Part model, mm, in its own coordinate system. Face numbers are marked on the shaded views. A direction names the side the tool comes from. Give positions to 0.01 mm unless a question says otherwise; leave off trailing zeros. Order: outer loops, then holes, each group sorted by start corner. A loop starts at its lowest first (then second) coordinate and runs counter-clockwise, first axis right, second up.
1. Drop flat-ended pins along their axis: pin 1 Ø1.5 at (x, z) = (42, 3.5) entering from +Y; pin 2 Ø2.5 at (y, z) = (64.5, 93.5) entering from -X; pin 3 Ø3 at (y, z) = (50, 36) entering from +X. Give the stop position or say it passes through.
2. Slice it at B-B on x = 56. List the corners of the cut face in (y, z), and give its area (3 significant figures).
3. Which spindle directions (+Z, -Z, +X, -X, +Y, -Y) get a long thin tool onto all of the face, cutting with end or side? Do the marked faces 4, 5 and 6. Say none if no direction does.
4. Probe line 1 (Z direction, x = 44.5, y = 51.5); line 2 (X direction, y = 27, z = 35). List the from-to ranges inside material, lowest first.
5. Slice it at C-C on z = 46.5. List the corners of the cut face in (x, y), and give its area (3 significant figures).
6. Slice it at D-D on y = 27. List the corners of the cut face in (x, z).
7. Mould opens along Z. For the marked faces 1, 2 and 3 say: +Z half, -Z half, draft (parallel to the pull), parting line (faces both ways), or undercut.
8. Slice it at A-A on y = 58. List the corners of the cut face in (x, z).
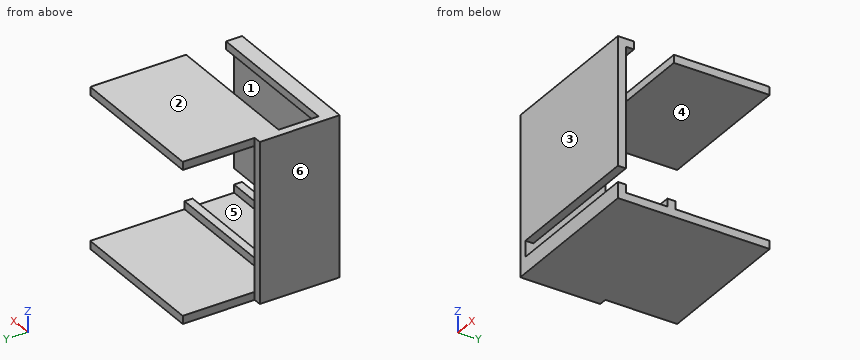
from build123d import *

# Parameters (mm, degrees)
F3_W     = 50
F3_H     = 100
F4_DEPTH = 5
F0_W     = 5
F0_H     = 5
F2_W     = 60
F2_H     = 5
F5_DEPTH = 90
F6_ANGLE = 90
F7_ANGLE = 90


with BuildPart() as f4:
    # F3 (on Top) → F4 (new body)
    with BuildSketch(Plane.XY):
        with Locations((25, 50)):
            Rectangle(F3_W, F3_H)
    extrude(amount=-F4_DEPTH)

    # F0 (on Top) + F1 (on Top) + F2 (on Top) → F5 (join)
    with BuildSketch(Plane.XY):
        Polygon((0, 10), (0, 0), (95, 0), (95, 5), (36, 5), (31, 5), (5, 5), (5, 10), align=None)
        with Locations((33.5, 7.5)):
            Rectangle(F0_W, F0_H)
    with BuildSketch(Plane.XY):
        Polygon((0, 100), (0, 20), (5, 20), (5, 95), (10, 95), (10, 100), align=None)
    with BuildSketch(Plane.XY):
        with Locations((65, 97.5)):
            Rectangle(F2_W, F2_H)
    extrude(amount=F5_DEPTH)


with BuildPart() as f4_1:
    # F6: moved
    add(f4.part.rotate(Axis((25, 0, -5), (1, 0, 0)), F6_ANGLE))


with BuildPart() as f4_2:
    # F7: moved
    add(f4_1.part.rotate(Axis((0, 0, 45), (0, 0, 1)), F7_ANGLE))


solid = f4_2.part
Data:
1. pin 1: stops at y = 36
1. pin 2: stops at x = 5
1. pin 3: stops at x = 5
2. outline: (0, -5) - (95, -5) - (95, 0) - (36, 0) - (36, 5) - (31, 5) - (31, 0) - (5, 0) - (5, 5) - (0, 5) - close; (0, 15) - (5, 15) - (5, 90) - (10, 90) - (10, 95) - (0, 95) - close; (35, 90) - (95, 90) - (95, 95) - (35, 95) - close
2. area: 1,250 mm2
3. face 4: +X, +Y
3. face 5: +X
3. face 6: +Z, -Z, -X, +Y, -Y
4. line 1: z = -5 to 0, 90 to 95
4. line 2: x = 0 to 5
5. outline: (0, 0) - (95, 0) - (95, 5) - (5, 5) - (5, 50) - (0, 50) - close
5. area: 700 mm2
6. outline: (0, -5) - (95, -5) - (95, 0) - (5, 0) - (5, 95) - (0, 95) - close
7. face 1: undercut
7. face 2: +Z half
7. face 3: draft
8. outline: (5, -5) - (95, -5) - (95, 0) - (5, 0) - close; (5, 90) - (95, 90) - (95, 95) - (5, 95) - close
